```python
from build123d import *

# Parameters (mm, degrees)
SKETCH1_W                   = 24
SKETCH1_H                   = 14
BOSS_EXTRUDE1_DEPTH         = 3
F_44_0_086_DIAMETER_HOLE3_D = 2.1844
SKETCH6_W                   = 3.1
SKETCH6_H                   = 6
SKETCH6_W_2                 = 5.4
SKETCH6_H_2                 = 2.2
CUT_EXTRUDE1_DEPTH          = 3


with BuildPart() as part:
    # Sketch1 → Boss-Extrude1 (new body)
    with BuildSketch(Plane(origin=(0, 0, 0), x_dir=(0, 0, -1), z_dir=(1, 0, 0))):
        with Locations((12, 7)):
            Rectangle(SKETCH1_W, SKETCH1_H)
    extrude(amount=BOSS_EXTRUDE1_DEPTH)

    # #44 (0.086) Diameter Hole3 (through all)
    with Locations(Plane(origin=(3, 0, 0), x_dir=(0, 0, -1), z_dir=(1, 0, 0))):
        with Locations((3.11, 11.05), (20.889999972, 11.049), (20.889999944, 2.159), (3.11, 2.16)):
            Hole(F_44_0_086_DIAMETER_HOLE3_D / 2)

    # Sketch6 → Cut-Extrude1 (cut)
    with BuildSketch(Plane(origin=(3, 0, 0), x_dir=(0, 0, -1), z_dir=(1, 0, 0))):
        with Locations((12, 11)):
            Rectangle(SKETCH6_W, SKETCH6_H)
        with Locations((12, 11.1)):
            Rectangle(SKETCH6_W_2, SKETCH6_H_2)
    extrude(amount=-CUT_EXTRUDE1_DEPTH, mode=Mode.SUBTRACT)


solid = part.part
```
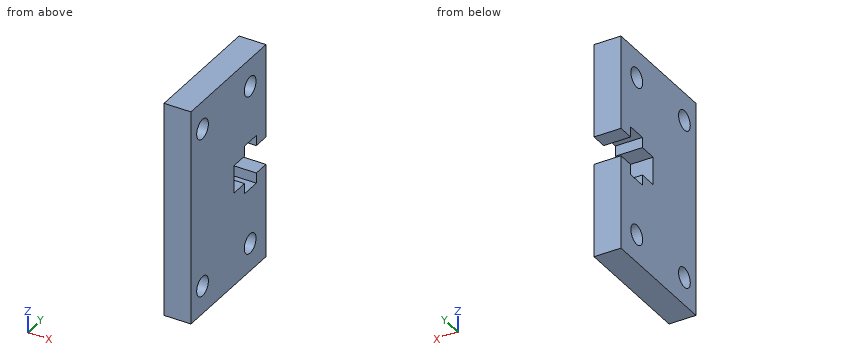
Geometry check sheet. Reference: the model listing, model coordinates, mm. Give positions to 0.01 mm unless a question says otherwise; leave off trailing zeros. Write each loop counter-clockwise with the first axis right and the second up, starting at its lowest first coordinate (ties: lowest second). Pieces come first, ordered by that corner, then holes.
1) Section check D-D, the plane z = -2.5. Record the boundary of the cut face in (x, y), and give its area (3 significant figures).
2) Section check A-A, the plane z = -20.89. Record the boundary of the cut face in (x, y).
3) Section check C-C, the plane y = 10.25. Record the boundary of the cut face in (x, z).
4) Gauge pin test, flat end, axial feed: pin 1 (1.5 mm diameter, centred on x = 2, z = -12.5, fed in from +Y). Record the tip position at first contact, or that the pin passes through.
5) Section check B-B, the plane x = 1.75. Record the boundary of the cut face in (y, z), and give its area (3 significant figures).
6) Material ranges on L1, parallel to Y at x = 0.7, z = -3.11; L2, parallel to Z at x = 0.45, y = 9; L3, parallel to Y at x = 0.4, z = -14, recorded low to high.
Computed:
1. outline: (0, 0) - (3, 0) - (3, 1.25) - (0, 1.25) - close; (0, 3.07) - (3, 3.07) - (3, 10.14) - (0, 10.14) - close; (0, 11.96) - (3, 11.96) - (3, 14) - (0, 14) - close
1. area: 31.1 mm2
2. outline: (0, 0) - (3, 0) - (3, 1.07) - (0, 1.07) - close; (0, 3.25) - (3, 3.25) - (3, 9.96) - (0, 9.96) - close; (0, 12.14) - (3, 12.14) - (3, 14) - (0, 14) - close
3. outline: (0, -24) - (3, -24) - (3, -21.63) - (0, -21.63) - close; (0, -20.15) - (3, -20.15) - (3, -14.7) - (0, -14.7) - close; (0, -9.3) - (3, -9.3) - (3, -3.85) - (0, -3.85) - close; (0, -2.37) - (3, -2.37) - (3, 0) - (0, 0) - close
4. pin 1: stops at y = 8
5. outline: (0, -24) - (14, -24) - (14, -13.55) - (12.2, -13.55) - (12.2, -14.7) - (10, -14.7) - (10, -13.55) - (8, -13.55) - (8, -10.45) - (10, -10.45) - (10, -9.3) - (12.2, -9.3) - (12.2, -10.45) - (14, -10.45) - (14, 0) - (0, 0) - close; hole circle Ø2.18 at (2.16, -20.89); hole circle Ø2.18 at (2.16, -3.11); hole circle Ø2.18 at (11.05, -20.89); hole circle Ø2.18 at (11.05, -3.11)
5. area: 297 mm2
6. L1: y = 0 to 1.07, 3.25 to 9.96, 12.14 to 14
6. L2: z = -24 to -13.55, -10.45 to 0
6. L3: y = 0 to 10, 12.2 to 14
